Geometry: final body of the model. Coordinates: model frame, mm. A direction names the side the tool comes from. Give positions to 0.01 mm unless a question says otherwise; leave off trailing zeros. Loops run counter-clockwise (first coordinate to the right, second up) from the corner with the lowest first, then second, coordinate; pieces in that order, holes last. Notation, with made-up numbers: (2.25, 3) -> (8.25, 3) arc R36 cw to (8.25, 38) -> close; hole circle Ø3 at (65.25, 6). An arc over 180 degrees is marked (long way). Answer in a Markdown table with one row per item. Add a question column.
Autodesk Inventor part; units mm, degrees
ref_plane "YZ Plane" through (0, 0, 0) normal (1, 0, 0) x (0, 1, 0)
ref_plane "XZ Plane" through (0, 0, 0) normal (0, 1, 0) x (-1, 0, 0)
ref_plane "XY Plane" through (0, 0, 0) normal (0, 0, 1) x (1, 0, 0)
sketch "puzzle" plane through (0, 0, 0) normal (0, 1, 0) x (-1, 0, 0)
  line L0 (0, 0) -> (-150, 0)
  line L1 (0, -115) -> (-15, -115)
  line L2 (-135, -115) -> (-125, -115)
  line L3 (-135, -115) -> (-150, -115)
  line L4 (-75, -115) -> (-65, -115)
  line L5 (-75, -115) -> (-85.0002, -115)
  line L6 (-105, -135) -> (-94.9796, -135)
  line L7 (-94.9796, -135) -> (-115, -135)
  line L8 (-65, -115) -> (-60, -115)
  line L9 (-60, -125) -> (-63, -125)
  arc A0 (-60, -125) -> (-60, -115) centre (-60, -120) ccw
  arc A1 (-63, -125) -> (-63, -135) centre (-63, -130) ccw
  line L10 (-85.0002, -115) -> (-90.0002, -115)
  line L11 (-94.9796, -135) -> (-89.9796, -135)
  arc A2 (-90.0002, -115) -> (-90, -125) centre (-90.0002, -120) ccw
  arc A3 (-89.9796, -135) -> (-90, -125) centre (-89.9796, -130) ccw
  line L12 (-115, -135) -> (-120, -135)
  line L13 (-125, -115) -> (-120, -115)
  arc A4 (-120, -125) -> (-120, -115) centre (-120, -120) ccw
  arc A5 (-120, -125) -> (-120, -135) centre (-120, -130) ccw
  line L14 (0, -115) -> (-30, -115)
  line L15 (-63, -135) -> (-32.98, -135)
  line L16 (-32.98, -135) -> (-32, -135)
  line L17 (-30, -115) -> (-32, -115)
  arc A6 (-32, -115) -> (-32, -125) centre (-32, -120) ccw
  arc A7 (-32, -135) -> (-32, -125) centre (-32, -130) ccw
  line L18 (-150, -115) -> (-150, 0)
  line L19 (0, -115) -> (0, 0)
  dimension "d22" = 5
  dimension "d23" = 5
  dimension "d24" = 5
  dimension "d25" = 5
  dimension "d26" = 5
extrude "Extrusión1" add sketch "puzzle" along normal blind 5
sketch "peus" plane through (0, 0, 0) normal (0, -1, 0) x (1, 0, 0)
  line L0 (150, 0) -> (145, 0)
  line L1 (150, 0) -> (100, 0)
  line L2 (0, -115) -> (0, 0)
  line L3 (0, 0) -> (50, 0)
  line L4 (50, 0) -> (50, -10)
  line L5 (0, 0) -> (10, 0)
  line L6 (10, -50) -> (0, -50)
  line L7 (0, -50) -> (0, 0)
  line L8 (50, -10) -> (10, -10)
  line L9 (10, -10) -> (10, -50)
  line L10 (100, 0) -> (100, -10)
  line L11 (100, -10) -> (140, -10)
  line L12 (140, -10) -> (140, -50)
  line L13 (140, -50) -> (150, -50)
  line L14 (150, 0) -> (150, -115)
  line L15 (150, 0) -> (150, -50)
  line L16 (0, 0) -> (150, 0)
  line L17 (45, -62.5) -> (45, -72.5)
  line L18 (105, -72.5) -> (105, -62.5)
  line L19 (80, -97.5) -> (70, -97.5)
  line L20 (80, -37.5) -> (70, -37.5)
  line L21 (80, -62.5) -> (70, -62.5)
  line L22 (70, -62.5) -> (70, -72.5)
  line L23 (70, -72.5) -> (80, -72.5)
  line L24 (80, -62.5) -> (80, -72.5)
  line L25 (83, -62.5) -> (83, -59.5)
  line L26 (83, -59.5) -> (80, -59.5)
  line L27 (70, -59.5) -> (67, -59.5)
  line L28 (67, -59.5) -> (67, -62.5)
  line L29 (67, -72.5) -> (67, -75.5)
  line L30 (67, -75.5) -> (70, -75.5)
  line L31 (80, -75.5) -> (83, -75.5)
  line L32 (83, -75.5) -> (83, -72.5)
  line L33 (83, -72.5) -> (105, -72.5)
  line L34 (83, -62.5) -> (105, -62.5)
  line L35 (80, -59.5) -> (80, -37.5)
  line L36 (70, -59.5) -> (70, -37.5)
  line L37 (67, -62.5) -> (45, -62.5)
  line L38 (67, -72.5) -> (45, -72.5)
  line L39 (70, -75.5) -> (70, -97.5)
  line L40 (80, -75.5) -> (80, -97.5)
  line L41 (83, -72.5) -> (105, -72.5)
  dimension "d70" = 3
extrude "Extrusión3" add sketch "peus" along normal blind 25
sketch "Boceto4" plane through (0, 0, 0) normal (0, -1, 0) x (1, 0, 0)
  line L0 (55, -135) -> (37, -135)
  line L1 (120, -135) -> (89.9796, -135)
  line L2 (115, -135) -> (95, -135)
  line L3 (90.0002, -115) -> (60, -115)
  line L4 (75.0001, -115) -> (83.5001, -115)
  line L5 (83.5001, -115) -> (66.5001, -115)
  line L6 (83.5001, -110) -> (66.5001, -110)
  line L7 (83.5001, -110) -> (83.5001, -115)
  line L8 (66.5001, -110) -> (66.5001, -115)
  line L9 (55, -130) -> (37, -130)
  line L10 (55, -130) -> (55, -135)
  line L11 (37, -130) -> (37, -135)
  line L12 (115, -130) -> (95, -130)
  line L13 (95, -130) -> (95, -135)
  line L14 (115, -130) -> (115, -135)
  point P0 (0, 0)
extrude "Extrusión4" add sketch "Boceto4" along normal blind 10
sketch "Boceto5" plane through (55, 0, -135) normal (0, 0, -1) x (-1, 0, 0)
  circle A0 centre (9, -5) radius 1.6
  circle A1 centre (-50, -5) radius 1.6
  point P0 (55, 0)
  dimension "d81" = 3.2
  dimension "d82" = 3.2
extrude "Extrusión5" cut sketch "Boceto5" against normal blind 14.25
sketch "Boceto6" plane through (95, 0, -130) normal (0, 0, 1) x (1, 0, 0)
  circle A0 centre (-49, -5) radius 1.6
  circle A1 centre (-49, -5) radius 3.05
  circle A2 centre (10, -5) radius 1.6
  circle A3 centre (10, -5) radius 3.05
  point P0 (-95, 0)
  dimension "d85" = 6.1
  dimension "d86" = 6.1
extrude "Extrusión6" cut sketch "Boceto6" against normal blind 2
sketch "Boceto7" plane through (66.5001, 0, -110) normal (0, 0, 1) x (1, 0, 0)
  line L0 (17, -10) -> (0, -10)
  line L1 (8.5, -10) -> (8.5, 0)
  line L2 (0, 0) -> (17, 0)
  circle A0 centre (8.5, -5) radius 3.05
  point P0 (-66.5001, 0)
  dimension "d89" = 6.1
extrude "Extrusión7" cut sketch "Boceto7" against normal blind 2
sketch "Boceto8" plane through (66.5001, 0, -110) normal (0, 0, 1) x (1, 0, 0)
  circle A0 centre (8.5, -5) radius 3.05
  circle A1 centre (8.5, -5) radius 1.6
  point P0 (-66.5001, 0)
  dimension "d92" = 3.2
extrude "Extrusión8" cut sketch "Boceto8" against normal blind 13 contours A1
sketch "Boceto9" plane through (140, 0, -50) normal (-1, 0, 0) x (0, 0, 1)
  line L0 (0, 0) -> (0, -25)
  line L1 (0, -25) -> (40, -25)
  line L2 (40, -25) -> (0, -25)
  line L3 (0, 0) -> (40, 0)
  line L4 (0, 0) -> (0, -25)
  line L5 (0, -25) -> (15, -25)
  line L6 (15, -25) -> (15, 0)
  line L7 (15, -25) -> (30, -25)
  line L8 (30, -25) -> (30, 0)
  circle A0 centre (15, -12.5) radius 1.7
  circle A1 centre (30, -12.5) radius 1.7
  point P0 (50, 0)
  dimension "d96" = 15
  dimension "d97" = 15
  dimension "d98" = 3.4
  dimension "d99" = 3.4
extrude "Extrusión9" cut sketch "Boceto9" against normal blind 19.75 contours A0 L6 | L6 A0 | A1 L8 | L8 A1
properties part number "base auxiliar 1"
(1) Draft query along X for faces 4 (the cylindrical face through (68, 2, -130)), 5 (the flat face through (5, -12, -50)), 6 (the flat face through (105, -12, -68)), 7 (the flat face through (70, -12, -86)). Return one class per face: +X half, -X half, draft (parallel to the pull), parting line (faces both ways), or undercut.
(2) Cut plane C-C on x = 15.5. Return the cut outline in (y, z).
(3) Cut plane B-B on z = -66.5. Return the cut outline in (x, y).
(4) Cut plane D-D on y = 1.75. Return the cut outline in (x, z), then the cut area to 3 significant figures.
(5) Cut plane A-A on z = -120. Return the cut outline in (x, y), then the cut area to 3 significant figures.
(6) Pin query (flat end, axial travel): pin 1 Ø11 at (x, y) = (72.5, -11.5) entering from -Z; pin 2 Ø2.5 at (y, z) = (-5.5, -111.5) entering from +X; pin 3 Ø1.5 at (x, z) = (75.5, -111) entering from -Y. Return the tip coordinate at first contact, or that it passes through.
(7) Material intervals for line 1 along Z through (x, y) = (143, -12.5); line 2 along X through (y, z) = (-5, -134.2); line 3 along X through (y, z) = (-18.75, -15.5), sorted ascending. Write a range as from..to.
(8) Reachability of faces 1 (the cylindrical face through (76.526, -4.519, -113.479)), 2 (the flat face through (120, -12, -10)), 3 (the flat face through (55, -5, -132)) from +Z, -Z, +X, -X, +Y, -Y: full face, straight path, thin tool, end or side. Return the list, or none.
Answer list:
| question | item | result |
|---|---|---|
| 1 | face 4 | undercut |
| 1 | face 5 | draft |
| 1 | face 6 | +X half |
| 1 | face 7 | -X half |
| 2 | outline | (-25, -10) -> (0, -10) -> (0, -115) -> (5, -115) -> (5, 0) -> (-25, 0) -> close |
| 3 | outline | (0, 0) -> (45, 0) -> (45, -25) -> (70, -25) -> (70, 0) -> (80, 0) -> (80, -25) -> (105, -25) -> (105, 0) -> (150, 0) -> (150, 5) -> (0, 5) -> close |
| 4 | outline | (0, -115) -> (32, -115) arc R5 cw to (32, -125) arc R5 ccw to (32, -135) -> (63, -135) arc R5 ccw to (63, -125) -> (60, -125) arc R5 cw to (60, -115) -> (90, -115) arc R5 cw to (90, -125) arc R5 ccw to (89.98, -135) -> (120, -135) arc R5 ccw to (120, -125) arc R5 cw to (120, -115) -> (150, -115) -> (150, 0) -> (0, 0) -> close |
| 4 | area | 18,400 mm² |
| 5 | outline | (37, 0) -> (55, 0) -> (55, 5) -> (37, 5) -> close; (95, 0) -> (115, 0) -> (115, 5) -> (95, 5) -> close |
| 5 | area | 190 mm² |
| 6 | pin 1 | stops at z = -115 |
| 6 | pin 2 | stops at x = 83.5 |
| 6 | pin 3 | stops at y = -10 |
| 7 | line 1 | z = -50..-36.7, -33.3..-21.7, -18.3..0 |
| 7 | line 2 | x = 37..44.4, 47.6..55, 95..103.4, 106.6..115 |
| 7 | line 3 | x = 0..10, 140..150 |
| 8 | face 1 | -Z |
| 8 | face 2 | -Y |
| 8 | face 3 | -Z, -Y |
